Design review of the part built by this model. Coordinates are the model's own, in mm. Coordinates: 2 decimals unless noted, no trailing zeros. Answer as a JSON object with one key per item and string values. Group by question number.
1. Insertion check: pin 1 (2 mm diameter, centred on y = 448, z = 32.5, fed in from -X). The pin has a flat end and moves straight along its axis. Give the tip position at first contact, or say it passes through.
2. Consider section B-B (x = 101.6). Count the separate pieces of the cut face and the enclosed holes in it, then the cut area to 3 significant figures.
3. Draft analysis for pull direction Y (two halves, no side actions). For faces 1 (the cylindrical face through (97.98, 85.297, 18.783)), 2 (the flat face through (108, 660.4, 20)), 3 (the flat face through (110, 335, 38.1)), 4 (the cylindrical face through (99.43, 575.36, 18.78)), state which applies: +Y half, -Y half, draft (parallel to the pull), parting line (faces both ways), or undercut.
4. To check wall thickness, follow probe 1 along Y at (x, z) = (101.6, 29); probe 2 along X at (y, z) = (390.5, 34); probe 3 along X at (y, z) = (429.5, 35.5). State the ranges of each line that lie inside material, in increasing order.
from build123d import *

# Parameters (mm, degrees)
F0_W     = 215.9
F0_H     = 660.4
F0_R     = 16.7005
F1_DEPTH = 38.1
F2_SIZE  = 6.35
F3_R     = 3.175


with BuildPart() as f1:
    # F0 (on Top) → F1 (new body)
    with BuildSketch(Plane.XY):
        with Locations((107.95, 330.2)):
            Rectangle(F0_W, F0_H)
        with Locations((101.6, 101.6)):
            Circle(F0_R, mode=Mode.SUBTRACT)
        with Locations((101.6, 558.8)):
            Circle(F0_R, mode=Mode.SUBTRACT)
    extrude(amount=F1_DEPTH)

    # F2
    f2_edges = [f1.edges().sort_by_distance(p)[0] for p in [
        (0, 330.2, 38.1),
    ]]
    chamfer(f2_edges, length=F2_SIZE)

    # F3
    f3_edges = [f1.edges().sort_by_distance(p)[0] for p in [
        (215.9, 330.2, 0),
        (107.95, 660.4, 0),
        (107.95, 0, 0),
        (0, 330.2, 0),
        (0, 0, 15.875),
        (0, 660.4, 15.875),
    ]]
    fillet(f3_edges, radius=F3_R)


solid = f1.part
Findings below:
{
 "1": {"pin 1": "stops at x = 0"},
 "2": {"separate pieces": "3", "enclosed holes": "0", "area": "22,600 mm^2"},
 "3": {"face 1": "undercut", "face 2": "+Y half", "face 3": "draft", "face 4": "undercut"},
 "4": {"probe 1": "y = 0 to 84.9, 118.3 to 542.1, 575.5 to 660.4", "probe 2": "x = 2.25 to 215.9", "probe 3": "x = 3.75 to 215.9"}
}
